The model under review builds one solid part; all positions refer to its coordinate system, in mm. Face numbers are marked on the shaded views. A direction names the side the tool comes from. Round coordinates to 2 decimals unless told otherwise and drop trailing zeros. Loops run counter-clockwise (first coordinate to the right, second up) from the corner with the lowest first, then second, coordinate; pieces in that order, holes last. Notation, with made-up numbers: M -12,21.5 L 43,21.5 A15 cw 43,39.5 Z; hole C 13.5,-22 d7. An arc over 180 degrees is marked long. One line per question, with ' | ' between items.
Autodesk Fusion 360 part; units mm, degrees
sketch "Sketch1" plane through (0, 0, 0) normal (0, 1, 0) x (1, 0, 0)
  circle A0 centre (0, 0) radius 25.4
  dimension "d1" = 50.8
extrude "Extrude1" add sketch "Sketch1" along normal blind 12.7
sketch "Sketch2" plane through (0, 12.7, 0) normal (0, 1, 0) x (-1, 0, 0)
  circle A0 centre (0, 0) radius 25.4
  circle A1 centre (0, -25.4) radius 6.35
  dimension "d4" = 12.7
extrude "Extrude2" cut sketch "Sketch2" against normal blind 6.35 contours A0 A1 | A0 A1 picked at (-1.9477, -23.4128) picked at (2.1308, -27.1585)
sketch "Sketch3" plane through (0, 12.7, 0) normal (0, 1, 0) x (-1, 0, 0)
  arc A0 (6.3002, -24.6062) -> (-6.3002, -24.6062) centre (0, -25.4) ccw
  arc A1 (6.3002, -24.6063) -> (-6.3002, -24.6062) centre (0, 0) ccw
  circle A2 centre (0, -10.795) radius 4.7625
  circle A3 centre (0, -10.795) radius 2.5527
  dimension "d7" = 9.525
  dimension "d8" = 10.795
  dimension "d9" = 5.1054
sketch "Sketch4" plane through (0, 0, 0) normal (1, 0, 0) x (0, 0, -1)
  line L0 (25.4, 0) -> (25.4, 6.35)
  line L1 (-25.4, 12.7) -> (-25.4, 0)
  line L2 (19.05, 6.35) -> (24.6062, 6.35)
  line L3 (25.4, 6.35) -> (22.225, 6.35)
  line L4 (22.225, 7.9375) -> (25.4, 7.9375)
  line L5 (25.4, 7.9375) -> (25.4, 6.35)
  line L6 (22.225, 7.9375) -> (22.225, 6.35)
  dimension "d12" = 3.175
  dimension "d13" = 1.5875
revolve "Revolve1" cut sketch "Sketch4" angle 360 about axis through (0, 1.75, 0) along (0, 1, 0)
sketch "Sketch5" plane through (0, 12.7, 0) normal (0, 1, 0) x (-1, 0, 0)
  arc A0 (6.3002, -24.6062) -> (-6.3002, -24.6062) centre (0, -25.4) ccw
  arc A1 (6.3002, -24.6063) -> (-6.3002, -24.6062) centre (0, 0) ccw
  line L0 (0, -19.05) -> (0, 0) construction
  line L1 (0, 0) -> (0, 19.05) construction
  circle A2 centre (0, 25.4) radius 6.35
  arc A3 (5.1095, -21.6297) -> (-5.1095, -21.6297) centre (0, 0) ccw
  line L2 (-12.7, 9.525) -> (12.7, 9.525)
  line L3 (12.7, 9.525) -> (12.7, -9.525)
  line L4 (12.7, -9.525) -> (-12.7, -9.525)
  line L5 (-12.7, -9.525) -> (-12.7, 9.525)
  line L6 (-12.7, 9.525) -> (12.7, -9.525) construction
  line L7 (12.7, 9.525) -> (-12.7, -9.525) construction
  circle A4 centre (0, 0) radius 15.875
  dimension "d15" = 25.4
  dimension "d16" = 19.05
  dimension "d17" = 31.75
extrude "Extrude4" add sketch "Sketch5" along normal blind 5.08 contours L2 L3 L4 L5
equation "d17 = d15 + 0.25 in"
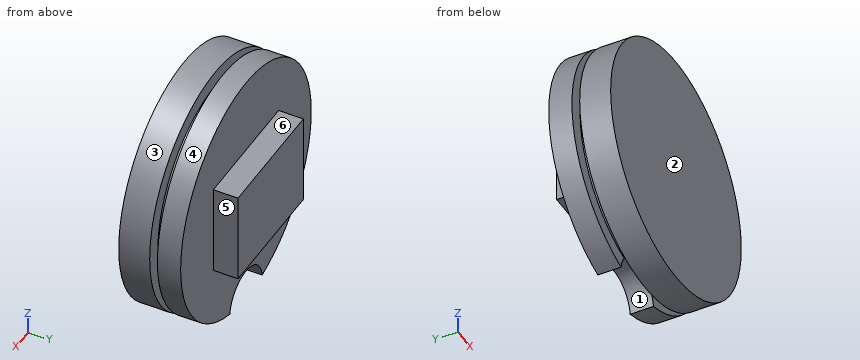
1) Insertion check: P1, Ø4, axis at x = 5, y = 16, coming from the +Z side (3 decimals); P2, Ø8, axis at y = 13.5, z = 9, coming from the -X side; P3, Ø1.5, axis at y = 14.5, z = -4, coming from the +X side. Each pin has a flat end and moves straight along its axis. Give the tip position at first contact, or say it passes through.
Output values:
P1: stops at z = 9.525 | P2: stops at x = -24.89 | P3: stops at x = 12.7
2) Add section D-D on z = 13. State the section outline as (x, y) points, then the cut area to 3 significant figures.
Output values:
outline: M -21.82,0 L 21.82,0 L 21.82,6.35 L 18.03,6.35 L 18.03,7.94 L 21.82,7.94 L 21.82,12.7 L -21.82,12.7 L -21.82,7.94 L -18.03,7.94 L -18.03,6.35 L -21.82,6.35 Z | area: 542 mm²
3) Machinability: for the marked faces 4, 5 and 6, which of the approach directions +Z, -Z, +X, -X, +Y, -Y give a long, thin tool a straight path to every point of the face, cutting with its end or side? Answer none if there is none.
Output values:
face 4: +Y, -Y | face 5: +Z, -Z, +X, +Y | face 6: +Z, +X, -X, +Y
4) Mouldability with a two-part tool opening along X and no side actions: class the marked faces 1, 2 and 3 as +X half, -X half, draft (parallel to the pull), parting line (faces both ways), or undercut.
Output values:
face 1: undercut | face 2: draft | face 3: parting line
5) For line 1 (Y direction, x = -16, z = -4); line 2 (Y direction, x = -22, z = 4.5); line 3 (X direction, y = 16.5, z = 5), list the stretches that pass through material, from the lowest coordinate up.
Output values:
line 1: y = 0 to 12.7 | line 2: y = 0 to 6.35, 7.94 to 12.7 | line 3: x = -12.7 to 12.7
6) Add section C-C on y = 16.25. State the section outline as (x, z) points (3 decimals).
Output values:
outline: M -12.7,-9.525 L 12.7,-9.525 L 12.7,9.525 L -12.7,9.525 Z
